For this review, take the finished solid that the model builds, in its own axes (mm). Face numbers are marked on the shaded views. Give positions to 0.01 mm unless a question says otherwise; leave off trailing zeros. Loops run counter-clockwise (first coordinate to the right, second up) from the corner with the lowest first, then second, coordinate; pieces in that order, holes last.
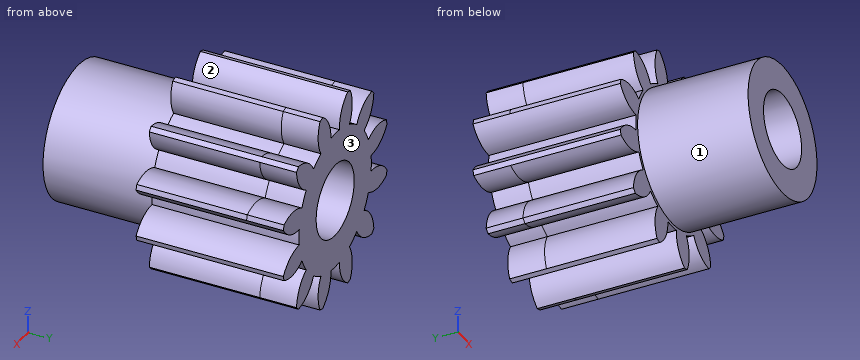
```python
from build123d import *

# Parameters (mm, degrees)
SKETCH1_R           = 17
BOSS_EXTRUDE1_DEPTH = 20
SKETCH2_R           = 17
CUT_EXTRUDE1_DEPTH  = 15
SKETCH4_R           = 17
CUT_EXTRUDE2_DEPTH  = 5
SKETCH5_R           = 9.05
BOSS_EXTRUDE2_DEPTH = 15
SKETCH6_R           = 5
CUT_EXTRUDE3_DEPTH  = 35


with BuildPart() as part:
    # Sketch1 → Boss-Extrude1 (new body)
    with BuildSketch(Plane(origin=(0, 0, 0), x_dir=(1, 0, 0), z_dir=(0, 1, 0))):
        Circle(SKETCH1_R)
    extrude(amount=BOSS_EXTRUDE1_DEPTH)

    # Sketch2 → Cut-Extrude1 (cut)
    with BuildSketch(Plane(origin=(-13.818246137, 15, -17.496579046), x_dir=(1, 0, 0), z_dir=(0, 1, 0))):
        with Locations((13.818246137, -17.496579046)):
            Circle(SKETCH2_R)
        with BuildLine():
            ThreePointArc((19.498036508, -25.110446812), (21.14436633, -26.898819817), (23.455733413, -27.651323701))
            ThreePointArc((23.455733413, -27.651323701), (23.717741074, -27.396073983), (23.972990792, -27.134066322))
            ThreePointArc((23.972990792, -27.134066322), (23.220486908, -24.822699239), (21.432113903, -23.176369417))
            ThreePointArc((21.432113903, -23.176369417), (22.044621448, -22.246079046), (22.544022769, -21.250486767))
            ThreePointArc((22.544022769, -21.250486767), (24.86397272, -21.97609831), (27.241927274, -21.472102249))
            ThreePointArc((27.241927274, -21.472102249), (27.341207705, -21.120045678), (27.431256615, -20.765515528))
            ThreePointArc((27.431256615, -20.765515528), (25.623885593, -19.140064859), (23.251944228, -18.608487912))
            ThreePointArc((23.251944228, -18.608487912), (23.317246137, -17.496579046), (23.251944228, -16.38467018))
            ThreePointArc((23.251944228, -16.38467018), (25.623885593, -15.853093234), (27.431256615, -14.227642564))
            ThreePointArc((27.431256615, -14.227642564), (27.341207705, -13.873112415), (27.241927274, -13.521055844))
            ThreePointArc((27.241927274, -13.521055844), (24.86397272, -13.017059783), (22.544022769, -13.742671325))
            ThreePointArc((22.544022769, -13.742671325), (22.044621448, -12.747079046), (21.432113903, -11.816788676))
            ThreePointArc((21.432113903, -11.816788676), (23.220486908, -10.170458854), (23.972990792, -7.85909177))
            ThreePointArc((23.972990792, -7.85909177), (23.717741074, -7.59708411), (23.455733413, -7.341834391))
            ThreePointArc((23.455733413, -7.341834391), (21.14436633, -8.094338276), (19.498036508, -9.882711281))
            ThreePointArc((19.498036508, -9.882711281), (18.567746137, -9.270203736), (17.572153858, -8.770802415))
            ThreePointArc((17.572153858, -8.770802415), (18.297765401, -6.450852463), (17.79376934, -4.072897909))
            ThreePointArc((17.79376934, -4.072897909), (17.441712769, -3.973617478), (17.087182619, -3.883568568))
            ThreePointArc((17.087182619, -3.883568568), (15.46173195, -5.69093959), (14.930155003, -8.062880955))
            ThreePointArc((14.930155003, -8.062880955), (13.818246137, -7.997579046), (12.706337271, -8.062880955))
            ThreePointArc((12.706337271, -8.062880955), (12.174760325, -5.69093959), (10.549309655, -3.883568568))
            ThreePointArc((10.549309655, -3.883568568), (10.194779506, -3.973617478), (9.842722935, -4.072897909))
            ThreePointArc((9.842722935, -4.072897909), (9.338726874, -6.450852463), (10.064338416, -8.770802415))
            ThreePointArc((10.064338416, -8.770802415), (9.068746137, -9.270203736), (8.138455767, -9.882711281))
            ThreePointArc((8.138455767, -9.882711281), (6.492125945, -8.094338276), (4.180758862, -7.341834391))
            ThreePointArc((4.180758862, -7.341834391), (3.918751201, -7.59708411), (3.663501482, -7.85909177))
            ThreePointArc((3.663501482, -7.85909177), (4.416005367, -10.170458854), (6.204378372, -11.816788676))
            ThreePointArc((6.204378372, -11.816788676), (5.591870827, -12.747079046), (5.092469506, -13.742671325))
            ThreePointArc((5.092469506, -13.742671325), (2.772519554, -13.017059783), (0.394565, -13.521055844))
            ThreePointArc((0.394565, -13.521055844), (0.295284569, -13.873112415), (0.205235659, -14.227642564))
            ThreePointArc((0.205235659, -14.227642564), (2.012606681, -15.853093234), (4.384548046, -16.38467018))
            ThreePointArc((4.384548046, -16.38467018), (4.319246137, -17.496579046), (4.384548046, -18.608487912))
            ThreePointArc((4.384548046, -18.608487912), (2.012606681, -19.140064859), (0.205235659, -20.765515528))
            ThreePointArc((0.205235659, -20.765515528), (0.295284569, -21.120045678), (0.394565, -21.472102249))
            ThreePointArc((0.394565, -21.472102249), (2.772519554, -21.97609831), (5.092469506, -21.250486767))
            ThreePointArc((5.092469506, -21.250486767), (5.591870827, -22.246079046), (6.204378372, -23.176369417))
            ThreePointArc((6.204378372, -23.176369417), (4.416005367, -24.822699239), (3.663501482, -27.134066322))
            ThreePointArc((3.663501482, -27.134066322), (3.918751201, -27.396073983), (4.180758862, -27.651323701))
            ThreePointArc((4.180758862, -27.651323701), (6.492125945, -26.898819817), (8.138455767, -25.110446812))
            ThreePointArc((8.138455767, -25.110446812), (9.068746137, -25.722954357), (10.064338416, -26.222355678))
            ThreePointArc((10.064338416, -26.222355678), (9.338726874, -28.542305629), (9.842722935, -30.920260183))
            ThreePointArc((9.842722935, -30.920260183), (10.194779506, -31.019540614), (10.549309655, -31.109589524))
            ThreePointArc((10.549309655, -31.109589524), (12.174760325, -29.302218502), (12.706337271, -26.930277137))
            ThreePointArc((12.706337271, -26.930277137), (13.818246137, -26.995579046), (14.930155003, -26.930277137))
            ThreePointArc((14.930155003, -26.930277137), (15.46173195, -29.302218502), (17.087182619, -31.109589524))
            ThreePointArc((17.087182619, -31.109589524), (17.441712769, -31.019540614), (17.79376934, -30.920260183))
            ThreePointArc((17.79376934, -30.920260183), (18.297765401, -28.542305629), (17.572153858, -26.222355678))
            ThreePointArc((17.572153858, -26.222355678), (18.567746137, -25.722954357), (19.498036508, -25.110446812))
        make_face(mode=Mode.SUBTRACT)
    extrude(amount=-CUT_EXTRUDE1_DEPTH, mode=Mode.SUBTRACT)

    # Sketch4 → Cut-Extrude2 (cut)
    with BuildSketch(Plane.XZ.offset(-15)):
        Circle(SKETCH4_R)
        with BuildLine():
            ThreePointArc((5.67979037, 7.613867765), (4.7495, 8.226375311), (3.753907721, 8.725776632))
            ThreePointArc((3.753907721, 8.725776632), (4.479519264, 11.045726583), (3.975523202, 13.423681137))
            ThreePointArc((3.975523202, 13.423681137), (3.623466631, 13.522961568), (3.268936482, 13.613010478))
            ThreePointArc((3.268936482, 13.613010478), (1.643485813, 11.805639456), (1.111908866, 9.433698091))
            ThreePointArc((1.111908866, 9.433698091), (0, 9.499), (-1.111908866, 9.433698091))
            ThreePointArc((-1.111908866, 9.433698091), (-1.643485813, 11.805639456), (-3.268936482, 13.613010478))
            ThreePointArc((-3.268936482, 13.613010478), (-3.623466631, 13.522961568), (-3.975523202, 13.423681137))
            ThreePointArc((-3.975523202, 13.423681137), (-4.479519264, 11.045726583), (-3.753907721, 8.725776632))
            ThreePointArc((-3.753907721, 8.725776632), (-4.7495, 8.226375311), (-5.67979037, 7.613867765))
            ThreePointArc((-5.67979037, 7.613867765), (-7.326120193, 9.402240771), (-9.637487276, 10.154744655))
            ThreePointArc((-9.637487276, 10.154744655), (-9.899494937, 9.899494937), (-10.154744655, 9.637487276))
            ThreePointArc((-10.154744655, 9.637487276), (-9.402240771, 7.326120193), (-7.613867765, 5.67979037))
            ThreePointArc((-7.613867765, 5.67979037), (-8.226375311, 4.7495), (-8.725776632, 3.753907721))
            ThreePointArc((-8.725776632, 3.753907721), (-11.045726583, 4.479519264), (-13.423681137, 3.975523202))
            ThreePointArc((-13.423681137, 3.975523202), (-13.522961568, 3.623466631), (-13.613010478, 3.268936482))
            ThreePointArc((-13.613010478, 3.268936482), (-11.805639456, 1.643485813), (-9.433698091, 1.111908866))
            ThreePointArc((-9.433698091, 1.111908866), (-9.499, 0), (-9.433698091, -1.111908866))
            ThreePointArc((-9.433698091, -1.111908866), (-11.805639456, -1.643485813), (-13.613010478, -3.268936482))
            ThreePointArc((-13.613010478, -3.268936482), (-13.522961568, -3.623466631), (-13.423681137, -3.975523202))
            ThreePointArc((-13.423681137, -3.975523202), (-11.045726583, -4.479519264), (-8.725776632, -3.753907721))
            ThreePointArc((-8.725776632, -3.753907721), (-8.226375311, -4.7495), (-7.613867765, -5.67979037))
            ThreePointArc((-7.613867765, -5.67979037), (-9.402240771, -7.326120193), (-10.154744655, -9.637487276))
            ThreePointArc((-10.154744655, -9.637487276), (-9.899494937, -9.899494937), (-9.637487276, -10.154744655))
            ThreePointArc((-9.637487276, -10.154744655), (-7.326120193, -9.402240771), (-5.67979037, -7.613867765))
            ThreePointArc((-5.67979037, -7.613867765), (-4.7495, -8.226375311), (-3.753907721, -8.725776632))
            ThreePointArc((-3.753907721, -8.725776632), (-4.479519264, -11.045726583), (-3.975523202, -13.423681137))
            ThreePointArc((-3.975523202, -13.423681137), (-3.623466631, -13.522961568), (-3.268936482, -13.613010478))
            ThreePointArc((-3.268936482, -13.613010478), (-1.643485813, -11.805639456), (-1.111908866, -9.433698091))
            ThreePointArc((-1.111908866, -9.433698091), (0, -9.499), (1.111908866, -9.433698091))
            ThreePointArc((1.111908866, -9.433698091), (1.643485813, -11.805639456), (3.268936482, -13.613010478))
            ThreePointArc((3.268936482, -13.613010478), (3.623466631, -13.522961568), (3.975523202, -13.423681137))
            ThreePointArc((3.975523202, -13.423681137), (4.479519264, -11.045726583), (3.753907721, -8.725776632))
            ThreePointArc((3.753907721, -8.725776632), (4.7495, -8.226375311), (5.67979037, -7.613867765))
            ThreePointArc((5.67979037, -7.613867765), (7.326120193, -9.402240771), (9.637487276, -10.154744655))
            ThreePointArc((9.637487276, -10.154744655), (9.899494937, -9.899494937), (10.154744655, -9.637487276))
            ThreePointArc((10.154744655, -9.637487276), (9.402240771, -7.326120193), (7.613867765, -5.67979037))
            ThreePointArc((7.613867765, -5.67979037), (8.226375311, -4.7495), (8.725776632, -3.753907721))
            ThreePointArc((8.725776632, -3.753907721), (11.045726583, -4.479519264), (13.423681137, -3.975523202))
            ThreePointArc((13.423681137, -3.975523202), (13.522961568, -3.623466631), (13.613010478, -3.268936482))
            ThreePointArc((13.613010478, -3.268936482), (11.805639456, -1.643485813), (9.433698091, -1.111908866))
            ThreePointArc((9.433698091, -1.111908866), (9.499, 0), (9.433698091, 1.111908866))
            ThreePointArc((9.433698091, 1.111908866), (11.805639456, 1.643485813), (13.613010478, 3.268936482))
            ThreePointArc((13.613010478, 3.268936482), (13.522961568, 3.623466631), (13.423681137, 3.975523202))
            ThreePointArc((13.423681137, 3.975523202), (11.045726583, 4.479519264), (8.725776632, 3.753907721))
            ThreePointArc((8.725776632, 3.753907721), (8.226375311, 4.7495), (7.613867765, 5.67979037))
            ThreePointArc((7.613867765, 5.67979037), (9.402240771, 7.326120193), (10.154744655, 9.637487276))
            ThreePointArc((10.154744655, 9.637487276), (9.899494937, 9.899494937), (9.637487276, 10.154744655))
            ThreePointArc((9.637487276, 10.154744655), (7.326120193, 9.402240771), (5.67979037, 7.613867765))
        make_face(mode=Mode.SUBTRACT)
    extrude(amount=-CUT_EXTRUDE2_DEPTH, mode=Mode.SUBTRACT)

    # Sketch5 → Boss-Extrude2 (add)
    with BuildSketch(Plane.XZ):
        Circle(SKETCH5_R)
    extrude(amount=BOSS_EXTRUDE2_DEPTH)

    # Sketch6 → Cut-Extrude3 (cut)
    with BuildSketch(Plane.XZ.offset(15)):
        Circle(SKETCH6_R)
    extrude(amount=-CUT_EXTRUDE3_DEPTH, mode=Mode.SUBTRACT)


solid = part.part
```
Q1. Consider section C-C on x = -8.25. Give the boundary of the cut face in (y, z).
Answers:
outline: (-15, -3.72) - (0, -3.72) - (0, -4.71) - (20, -4.71) - (20, 4.71) - (0, 4.71) - (0, 3.72) - (-15, 3.72) - close; (0, -9.86) - (20, -9.86) - (20, -6.08) - (0, -6.08) - close; (0, 6.08) - (20, 6.08) - (20, 9.86) - (0, 9.86) - close
Q2. Consider section D-D on y = -6. Give the boundary of the cut face in (x, z), plus the area to 3 significant figures.
Answers:
outline: circle Ø18.1 at (0, 0); hole circle Ø10 at (0, 0)
area: 179 mm2
Q3. Consider section A-A on x = 0. Give the boundary of the cut face in (y, z).
Answers:
outline: (-15, -9.05) - (0, -9.05) - (0, -9.5) - (20, -9.5) - (20, -5) - (-15, -5) - close; (-15, 5) - (20, 5) - (20, 9.5) - (0, 9.5) - (0, 9.05) - (-15, 9.05) - close
Q4. Mouldability with a two-part tool opening along X and no side actions: class the marked faces 1, 2 and 3 as +X half, -X half, draft (parallel to the pull), parting line (faces both ways), or undercut.
Answers:
face 1: parting line
face 2: undercut
face 3: draft
Q5. For pin 1 Ø4 at (x, y) = (6, -4) entering from +Z; pin 2 Ø4 at (y, z) = (2.5, -10.5) entering from -X; pin 3 Ø1 at (x, z) = (-9.5, 4) entering from -Y, all flat-tipped, find the tip position at first contact; note any pin that passes through.
Answers:
pin 1: stops at z = 8.12
pin 2: stops at x = -10.15
pin 3: stops at y = 0
Q6. For probe 1 along X at (y, z) = (8, -8.5); probe 2 along Z at (x, y) = (0, 8); probe 3 along X at (y, z) = (6, -9), list the stretches that pass through material, from the lowest coordinate up.
Answers:
probe 1: x = -9.95 to -6.29, -4.24 to 4.24, 6.29 to 9.95
probe 2: z = -9.5 to -5, 5 to 9.5
probe 3: x = -10.07 to -6.79, -3.91 to 3.91, 6.79 to 10.07
Q7. Consider section B-B on z = 0. Give the boundary of the cut face in (x, y), plus the area to 3 significant figures.
Answers:
outline: (-9.5, 0) - (-9.05, 0) - (-9.05, -15) - (-5, -15) - (-5, 20) - (-9.5, 20) - close; (5, -15) - (9.05, -15) - (9.05, 0) - (9.5, 0) - (9.5, 20) - (5, 20) - close
area: 301 mm2
